Can you work these out from the model? Positions are in its coordinate system, mm. Face numbers are marked on the shaded views. A direction names the side the tool comes from. Give positions to 0.01 mm unless a question says otherwise; leave off trailing zeros. Loops run counter-clockwise (first coordinate to the right, second up) from the corner with the lowest first, then second, coordinate; pieces in that order, holes last. Notation, with made-up numbers: M -2,-15 L 12,-15 A9 ccw 12,-9 Z; hole C 17.25,47 d3. An arc over 180 degrees is marked long. Answer as a JSON object with one key per item and string values.
Autodesk Inventor part; units mm, degrees
ref_plane "YZ Plane" through (0, 0, 0) normal (1, 0, 0) x (0, 1, 0)
ref_plane "XZ Plane" through (0, 0, 0) normal (0, 1, 0) x (-1, 0, 0)
ref_plane "XY Plane" through (0, 0, 0) normal (0, 0, 1) x (1, 0, 0)
sketch "Esquisse1" plane through (0, 0, 0) normal (0, 1, 0) x (-1, 0, 0)
  line L0 (35, 35) -> (35, 14)
  line L1 (35, 14) -> (42, 10)
  line L2 (42, 10) -> (42, 0)
  line L3 (35, 35) -> (0, 0)
  line L4 (42, 0) -> (0, 0) construction
  line L5 (35, -35) -> (35, -14)
  line L6 (35, -14) -> (42, -10)
  line L7 (42, -10) -> (42, 0)
  line L8 (35, -35) -> (0, 0)
  line L9 (38.5, -12) -> (38.5, 12) construction
  circle A0 centre (38.5, 0) radius 2.15
  circle A1 centre (38.5, 6) radius 2.15
  circle A2 centre (38.5, -6) radius 2.15
  dimension "d0" = 90
  dimension "d1" = 70
  dimension "d4" = 6
  dimension "d11" = 6
  dimension "d16" = 4.3
  dimension "d17" = 20
  dimension "d18" = 4
  dimension "d19" = 7
extrude "Extrusion1" add sketch "Esquisse1" along normal blind 3
pattern_circular "Réseau circulaire1" count 4 over 360 about axis through (0, 0, 0) along (0, 1, 0) of "Extrusion1"
ref_plane "Plan de construction2" through (0, 0, -14) normal (1, 0, 0) x (0, 0, -1)
ref_plane "Plan de construction3" through (-14, 0, 0) normal (0, 0, -1) x (-1, 0, 0)
chamfer "Chanfrein1" distance 10 angle 45 4 edges at (-35, 1.5, -35) (-35, 1.5, 35) (35, 1.5, -35) (35, 1.5, 35)
sketch "Esquisse3" plane through (0, 0, 0) normal (0, -1, 0) x (1, 0, 0)
  circle A0 centre (0, 38.5) radius 2.15 construction
  circle A1 centre (6, 38.5) radius 2.15 construction
  circle A2 centre (-6, 38.5) radius 2.15 construction
  circle A3 centre (38.5, 6) radius 2.15 construction
  circle A4 centre (38.5, -6) radius 2.15 construction
  circle A5 centre (38.5, 0) radius 2.15 construction
  circle A6 centre (6, -38.5) radius 2.15 construction
  circle A7 centre (-6, -38.5) radius 2.15 construction
  circle A8 centre (0, -38.5) radius 2.15 construction
  circle A9 centre (-38.5, -6) radius 2.15 construction
  circle A10 centre (-38.5, 6) radius 2.15 construction
  circle A11 centre (-38.5, 0) radius 2.15 construction
  line L0 (-35, 25) -> (-35, 14) construction
  line L1 (-35, 14) -> (-42, 10) construction
  line L2 (-42, 10) -> (-42, -10) construction
  line L3 (-42, -10) -> (-35, -14) construction
  line L4 (-35, -14) -> (-35, -25) construction
  line L5 (-25, -35) -> (-14, -35) construction
  line L6 (-14, -35) -> (-10, -42) construction
  line L7 (-10, -42) -> (10, -42) construction
  line L8 (10, -42) -> (14, -35) construction
  line L9 (14, -35) -> (25, -35) construction
  line L10 (35, -25) -> (35, -14) construction
  line L11 (35, -14) -> (42, -10) construction
  line L12 (42, -10) -> (42, 10) construction
  line L13 (42, 10) -> (35, 14) construction
  line L14 (35, 14) -> (35, 25) construction
  line L15 (25, 35) -> (14, 35) construction
  line L16 (14, 35) -> (10, 42) construction
  line L17 (10, 42) -> (-10, 42) construction
  line L18 (-10, 42) -> (-14, 35) construction
  line L19 (-14, 35) -> (-25, 35) construction
  line L20 (-51.72, -12.8291) -> (-12.8291, -51.72)
  line L21 (-12.8291, -51.72) -> (-10, -42)
  line L22 (-42, -10) -> (-51.72, -12.8291)
  line L23 (-35, -14) -> (-42, -10)
  line L24 (-42, -10) -> (-35, -14)
  line L25 (-10, -42) -> (-14, -35)
  line L26 (-14, -35) -> (-10, -42)
  line L27 (25, 35) -> (35, 25)
  line L28 (-35, 25) -> (-25, 35)
  line L29 (-25, -35) -> (-35, -25)
  line L30 (35, -25) -> (25, -35)
  line L31 (-14, -35) -> (-35, -14)
  point P0 (0, 0)
  dimension "d32" = 135
  dimension "d33" = 55
extrude "Extrusion3" add sketch "Esquisse3" against normal blind 3
sketch "Esquisse4" plane through (-51.72, 0, -12.8291) normal (-0.7071, 0, -0.7071) x (-0.7071, 0, 0.7071)
  line L0 (0, 0) -> (-55, 0) construction
  line L1 (0, 0) -> (0, 3) construction
  line L2 (-55, 3) -> (0, 3) construction
  line L3 (-55, 0) -> (-55, 3) construction
  line L4 (0, 0) -> (-55, 0)
  line L5 (-55, 0) -> (-55, 24)
  line L6 (-55, 24) -> (0, 24)
  line L7 (0, 24) -> (0, 0)
  point P0 (-27.5, 0)
  dimension "d36" = 24
extrude "Extrusion4" add sketch "Esquisse4" along normal blind 3
sketch "Esquisse5" plane through (-53.8413, 0, -14.9504) normal (-0.7071, 0, -0.7071) x (-0.7071, 0, 0.7071)
  line L0 (-55, 0) -> (0, 0) construction
  line L1 (0, 0) -> (0, 24) construction
  line L2 (0, 24) -> (-55, 24) construction
  line L3 (-55, 24) -> (-55, 0) construction
  line L4 (0, 0) -> (0, 24) construction
  line L5 (0, 9.2801) -> (-55, 9.2801) construction
  circle A0 centre (-15.1412, 9.2801) radius 7.3571
  line L6 (-27.5, 0) -> (-27.5, 24) construction
  circle A1 centre (-39.8588, 9.2801) radius 7.3571
extrude "Extrusion5" cut sketch "Esquisse5" against normal blind 1
pattern_circular "Réseau circulaire2" count 4 over 360 about axis through (0, 0, 0) along (0, -1, 0) of "Extrusion3", "Extrusion4"
fillet "Congé1" radius 3 2 edges at (-34.3959, 0, 34.3959) (34.3959, 0, -34.3959)
sketch "Esquisse13" plane through (0, 3, 0) normal (0, 1, 0) x (1, 0, 0)
  line L0 (-10, -42) -> (10, -42) construction
  line L1 (10, -42) -> (12.8291, -51.72) construction
  line L2 (12.8291, -51.72) -> (51.72, -12.8291) construction
  line L3 (51.72, -12.8291) -> (42, -10) construction
  line L4 (42, -10) -> (42, 10) construction
  line L5 (42, 10) -> (51.72, 12.8291) construction
  line L6 (51.72, 12.8291) -> (12.8291, 51.72) construction
  line L7 (12.8291, 51.72) -> (10, 42) construction
  line L8 (10, 42) -> (-10, 42) construction
  line L9 (-10, 42) -> (-12.8291, 51.72) construction
  line L10 (-12.8291, 51.72) -> (-51.72, 12.8291) construction
  line L11 (-51.72, 12.8291) -> (-42, 10) construction
  line L12 (-42, 10) -> (-42, -10) construction
  line L13 (-42, -10) -> (-51.72, -12.8291) construction
  line L14 (-51.72, -12.8291) -> (-12.8291, -51.72) construction
  line L15 (-12.8291, -51.72) -> (-10, -42) construction
  circle A0 centre (0, -38.5) radius 2.15 construction
  circle A1 centre (6, -38.5) radius 2.15 construction
  circle A2 centre (-6, -38.5) radius 2.15 construction
  circle A3 centre (38.5, -6) radius 2.15 construction
  circle A4 centre (38.5, 6) radius 2.15 construction
  circle A5 centre (38.5, 0) radius 2.15 construction
  circle A6 centre (6, 38.5) radius 2.15 construction
  circle A7 centre (-6, 38.5) radius 2.15 construction
  circle A8 centre (0, 38.5) radius 2.15 construction
  circle A9 centre (-38.5, 6) radius 2.15 construction
  circle A10 centre (-38.5, -6) radius 2.15 construction
  circle A11 centre (-38.5, 0) radius 2.15 construction
  line L16 (10, -42) -> (-18, -42)
  line L17 (-18, -42) -> (-42, -18)
  line L18 (-42, -18) -> (-42, 10)
  line L19 (-42, -10) -> (-42, 10)
  line L20 (-42, 10) -> (-35, 10)
  line L21 (-35, 10) -> (-35, -17.9289)
  line L22 (-35, -17.9289) -> (-17.9289, -35)
  line L23 (-17.9289, -35) -> (10, -35)
  line L24 (10, -35) -> (10, -42)
  line L25 (-10, -42) -> (10, -42)
  dimension "d97" = 7
  dimension "d98" = 5
  dimension "d99" = 28
extrude "Extrusion11" cut sketch "Esquisse13" against normal blind 10 keep common part
properties part number "renfort"
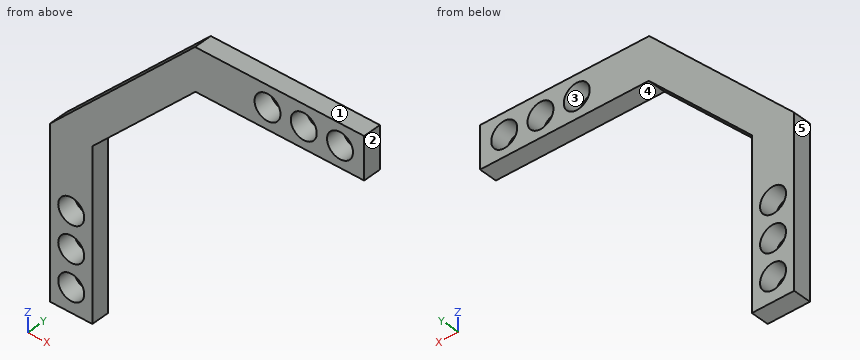
1) Suppose I cut it at C-C, the plane z = -6. Write out the boundary of the cut face in (x, y).
Answer list:
{"outline": "M -42,0 L -40.65,0 L -40.65,3 L -42,3 Z; M -36.35,0 L -35,0 L -35,3 L -36.35,3 Z"}
2) Suppose I cut it at B-B, the plane x = 0. Write out the boundary of the cut face in (y, z).
Answer list:
{"outline": "M 0,35 L 3,35 L 3,36.35 L 0,36.35 Z; M 0,40.65 L 3,40.65 L 3,42 L 0,42 Z"}
3) Will these pins go through, and if not, where does the flat tip stop? pin 1 Ø7 at (x, z) = (-38.5, 0) entering from -Y; pin 2 Ø1.5 at (y, z) = (2, 23) entering from +X.
Answer list:
{"pin 1": "y = 0", "pin 2": "x = -29.18"}
4) Suppose I cut it at A-A, the plane x = -38.5. Write out the boundary of the cut face in (y, z), and give its area (3 significant figures).
Answer list:
{"outline": "M 0,-10 L 3,-10 L 3,-8.15 L 0,-8.15 Z; M 0,-3.85 L 3,-3.85 L 3,-2.15 L 0,-2.15 Z; M 0,2.15 L 3,2.15 L 3,3.85 L 0,3.85 Z; M 0,8.15 L 3,8.15 L 3,21.5 L 0,21.5 Z", "area": "55.8 mm^2"}
5) If we mould it in two halves opening along X, with no side actions, what happens to the marked faces 1, 2 and 3? For each: +X half, -X half, draft (parallel to the pull), parting line (faces both ways), or undercut.
Answer list:
{"face 1": "draft", "face 2": "+X half", "face 3": "undercut"}
6) Suppose I cut it at D-D, the plane y = 0.95. Write out the boundary of the cut face in (x, z), and give its area (3 significant figures).
Answer list:
{"outline": "M -42,-10 L -35,-10 L -35,17.93 L -17.93,35 L 10,35 L 10,42 L -18,42 L -42,18 Z; hole C -38.5,-6 d4.3; hole C -38.5,0 d4.3; hole C -38.5,6 d4.3; hole C -6,38.5 d4.3; hole C 0,38.5 d4.3; hole C 6,38.5 d4.3", "area": "450 mm^2"}
7) For the marked faces 4 and 5, which set-ups out of +Z, -Z, +X, -X, +Y, -Y let a thin tool reach every point of the face, with its end or its side?
Answer list:
{"face 4": "-Z, +X, +Y, -Y", "face 5": "+Z, -Z, -X, +Y, -Y"}
8) Please list where these lines run through material, in increasing order: line 1 along X through (y, z) = (1.6, 38.5); line 2 along Z through (x, y) = (-38.5, 1.5); line 3 along X through (y, z) = (0.7, 6.5). Write a range as from..to.
Answer list:
{"line 1": "-21.5..-8.15, -3.85..-2.15, 2.15..3.85, 8.15..10", "line 2": "-10..-8.15, -3.85..-2.15, 2.15..3.85, 8.15..21.5", "line 3": "-42..-40.59, -36.41..-35"}
